Could you check a few things on this model? Use its own coordinates, in mm. Face numbers are marked on the shaded views. A direction names the side the tool comes from. Round coordinates to 2 decimals unless told otherwise and drop trailing zeros. Loops run counter-clockwise (first coordinate to the right, second up) from the corner with the lowest first, then second, coordinate; pieces in that order, holes last. Notation, with made-up numbers: M 62,70.25 L 114,70.25 A11 ccw 114,82.25 Z; hole C 31.25,27 d7. An arc over 180 degrees is marked long. One line per item, written item: value. Start each with the question number.
Q1. Please list where these lines run through material, in increasing order: line 1 along Z through (x, y) = (-1.62, 15.4); line 2 along Y through (x, z) = (-0.5, -5.5); line 3 along X through (y, z) = (18, -6.25).
Q2. Imagine slicing it at D-D (z = -7.25). Please give me the cut outline in (x, y), then the cut area to 3 significant figures.
Q3. Imagine slicing it at C-C (x = 16.5). Please give me the cut outline in (y, z), then the cut area to 3 significant figures.
Q4. Which directions (+Z, -Z, +X, -X, +Y, -Y) give clear straight access to the entire face, cutting with the end or side of a thin tool? Please do the marked faces 1, 2, 3 and 4.
Q5. Imagine slicing it at A-A (z = -4.3). Please give me the cut outline in (x, y).
Q6. I'm going to push flat-ended pins straight in: pin 1 Ø3 at (x, z) = (-2, -2.5) entering from +Y; pin 2 Ø4.5 at (y, z) = (6.5, -4) entering from +X; pin 3 Ø1.5 at (y, z) = (17, -2.5) entering from -X. Where does each tip first touch, or does it pass through?
Q7. Imagine slicing it at B-B (x = -1.62). Please give me the cut outline in (y, z), then the cut area to 3 significant figures.
from build123d import *

# Parameters (mm, degrees)
SKETCH_1_W          = 20.5
SKETCH_1_H          = 8.6
EXTRUDE_1_DEPTH     = 15.2
SKETCH_2_W          = 20.5
SKETCH_2_H          = 7.45
EXTRUDE_2_DEPTH     = 8.6
CHAMFER_1_SIZE      = 4
CHAMFER_1_SIZE2     = 11.616843511
SKETCH_3_W          = 3.5
SKETCH_3_H          = 1
EXTRUDE_3_DEPTH     = 8.6
SKETCH_4_R          = 0.8
CUT_EXTRUDE_1_DEPTH = 8.6
SKETCH_5_R          = 2
EXTRUDE_4_DEPTH     = 3


with BuildPart() as part:
    # 草图1 → 凸台-拉伸1 (new body)
    with BuildSketch(Plane(origin=(0, 0, 0), x_dir=(1, 0, 0), z_dir=(0, 1, 0))):
        with Locations((10.25, 4.3)):
            Rectangle(SKETCH_1_W, SKETCH_1_H)
    extrude(amount=EXTRUDE_1_DEPTH)

    # 草图2 → 凸台-拉伸2 (add)
    with BuildSketch(Plane.XY):
        with Locations((10.25, 18.925)):
            Rectangle(SKETCH_2_W, SKETCH_2_H)
    extrude(amount=-EXTRUDE_2_DEPTH)

    # 倒角1
    chamfer_1_edges = [part.edges().sort_by_distance(p)[0] for p in [
        (0, 22.65, -4.3),
    ]]
    chamfer_1_side = [part.faces().sort_by_distance(p)[0] for p in [
        (0, 11.325, -4.3),
    ]]
    chamfer(chamfer_1_edges, length=CHAMFER_1_SIZE, length2=CHAMFER_1_SIZE2, reference=chamfer_1_side[0])

    # 草图3 → 凸台-拉伸3 (add)
    with BuildSketch(Plane.XY):
        with Locations((-1.75, 15.2)):
            Rectangle(SKETCH_3_W, SKETCH_3_H)
        with Locations((22.25, 15.2)):
            Rectangle(SKETCH_3_W, SKETCH_3_H)
    extrude(amount=-EXTRUDE_3_DEPTH)

    # 草图4 → 切除-拉伸1 (cut)
    with BuildSketch(Plane(origin=(0, 15.7, 0), x_dir=(1, 0, 0), z_dir=(0, 1, 0))):
        with Locations(Location((-1.62, 4.3, 0), (0, 0, 180))):
            Circle(SKETCH_4_R)
        with Locations(Location((22.12, 4.3, 0), (0, 0, 180))):
            Circle(SKETCH_4_R)
    extrude(amount=-CUT_EXTRUDE_1_DEPTH, mode=Mode.SUBTRACT)

    # 草图5 → 凸台-拉伸4 (add)
    with BuildSketch(Plane(origin=(0, 22.65, 0), x_dir=(1, 0, 0), z_dir=(0, 1, 0))):
        with Locations(Location((16.5, 4.3, 0), (0, 0, 180))):
            Circle(SKETCH_5_R)
    extrude(amount=EXTRUDE_4_DEPTH)


solid = part.part
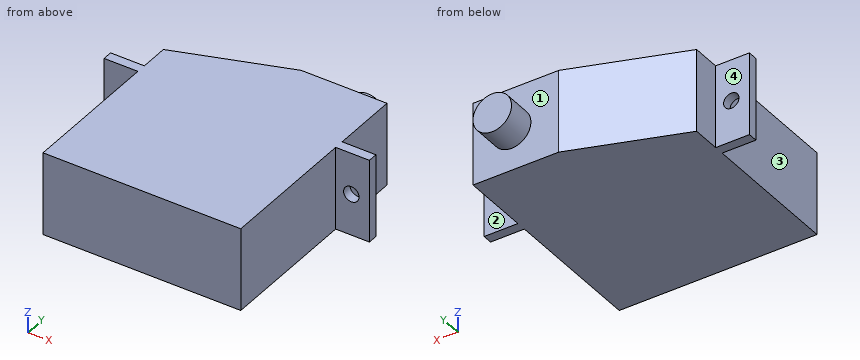
Report:
1. line 1: z = -8.6 to -5.1, -3.5 to 0
1. line 2: y = 14.7 to 15.7
1. line 3: x = 0 to 20.5
2. outline: M -3.5,14.7 L 0,14.7 L 0,0 L 20.5,0 L 20.5,14.7 L 24,14.7 L 24,15.7 L 20.5,15.7 L 20.5,22.65 L 11.62,22.65 L 0,18.65 L 0,15.7 L -3.5,15.7 Z
2. area: 448 mm²
3. outline: M 0,-8.6 L 22.65,-8.6 L 22.65,-6.3 L 25.65,-6.3 L 25.65,-2.3 L 22.65,-2.3 L 22.65,0 L 0,0 Z
3. area: 207 mm²
4. face 1: +Y
4. face 2: +Z, -Z, +X, +Y
4. face 3: +Z, -Z, -X, -Y
4. face 4: +Z, -Z, -X, +Y
5. outline: M -3.5,14.7 L -2.42,14.7 L -2.42,15.7 L -3.5,15.7 Z; M -0.82,14.7 L 0,14.7 L 0,0 L 20.5,0 L 20.5,14.7 L 21.32,14.7 L 21.32,15.7 L 20.5,15.7 L 20.5,22.65 L 18.5,22.65 L 18.5,25.65 L 14.5,25.65 L 14.5,22.65 L 11.62,22.65 L 0,18.65 L 0,15.7 L -0.82,15.7 Z; M 22.92,14.7 L 24,14.7 L 24,15.7 L 22.92,15.7 Z
6. pin 1: stops at y = 15.7
6. pin 2: stops at x = 20.5
6. pin 3: stops at x = 0
7. outline: M 14.7,-8.6 L 15.7,-8.6 L 15.7,-5.1 L 14.7,-5.1 Z; M 14.7,-3.5 L 15.7,-3.5 L 15.7,0 L 14.7,0 Z
7. area: 7.00 mm²
